Verification items for the finished model (mm, model axes). A direction names the side the tool comes from. Give positions to 0.01 mm unless a question says otherwise; leave off trailing zeros. Order: outer loops, then holes, each group sorted by start corner. A loop starts at its lowest first (then second) coordinate and runs counter-clockwise, first axis right, second up. Notation, with made-up numbers: (31, 68) -> (73, 68) arc R12 cw to (73, 82) -> close; hole circle Ø9 at (82.25, -28.75). An arc over 180 degrees is marked (long way). Return JSON: item names as keys, results as strings. Group by question number.
(1) Cross-section at C-C on y = -6.5. Enter the section's corners in (x, z), then the cut area to 3 significant figures.
(2) Thickness scan on line 1 along Z through (x, y) = (0, -2.25); line 2 along Y through (x, z) = (-5, 5); line 3 along Z through (x, y) = (2.5, -8). Record the ranges inside material, lowest first.
(3) Tool access check on faces 1 (the face through (11.9, -0.5, 2.5)), 2 (the face through (-11.8, -0.5, 2.5)), 3 (the face through (3, -1, 3)), 4 (the face through (11.9, -0.5, -2.5)). Record the directions out of +Z, -Z, +X, -X, +Y, -Y that give a thin tool (end or side, any length) a straight path to the whole face; none if there is none.
(4) Cross-section at A-A on x = 0. Enter the section's corners in (y, z).
(5) Cross-section at B-B on z = 0. Enter the section's corners in (x, y), then the cut area to 3 significant figures.
(6) Cross-section at D-D on z = -8.25. Enter the section's corners in (x, y), then the cut area to 3 significant figures.
(7) Depth check by flat-ended pin: pin 1 Ø4 at (x, y) = (-9, -4) entering from +Z; pin 2 Ø0.8 at (x, y) = (-11.5, -0.5) entering from -Z; pin 3 Ø3 at (y, z) = (-6, -3.5) entering from +X; pin 4 Ø3 at (y, z) = (-2, -8.5) entering from -X. Enter the tip coordinate at first touch or a pass-through.
from build123d import *

# Parameters (mm, degrees)
F0_R          = 11
F1_DEPTH      = 1
F3_W          = 26
F3_H          = 5
F4_DEPTH      = 1
F5_R          = 4
F5_R_2        = 3
F7_DEPTH      = 7.3
F6_R          = 3
F8_DEPTH      = 7.301
F8_DEPTH_BACK = 1.001


with BuildPart() as f1:
    # F0 (on Front) → F1 (new body)
    with BuildSketch(Plane.XZ):
        Circle(F0_R)
    extrude(amount=F1_DEPTH)

    # F3 (on face) → F4 (join)
    with BuildSketch(Plane(origin=(0, 0, 0), x_dir=(-1, 0, 0), z_dir=(0, 1, 0))):
        Rectangle(F3_W, F3_H)
    extrude(amount=-F4_DEPTH)

    # F5 (on face) → F7 (join)
    with BuildSketch(Plane.XZ.offset(1)):
        Circle(F5_R)
        Circle(F5_R_2, mode=Mode.SUBTRACT)
    extrude(amount=F7_DEPTH)

    # F6 (on face) → F8 (cut, two sides)
    with BuildSketch(Plane.XZ.offset(1)) as f8_sk:
        Circle(F6_R)
    extrude(amount=F8_DEPTH, mode=Mode.SUBTRACT)
    extrude(f8_sk.sketch, amount=-F8_DEPTH_BACK, mode=Mode.SUBTRACT)


solid = f1.part
Verdict:
{
 "1": {"outline": "circle Ø8 at (0, 0); hole circle Ø6 at (0, 0)", "area": "22.0 mm²"},
 "2": {"line 1": "-4 to -3, 3 to 4", "line 2": "-1 to 0", "line 3": "-3.12 to -1.66, 1.66 to 3.12"},
 "3": {"face 1": "+Z, +X, +Y, -Y", "face 2": "+Z, -X, +Y, -Y", "face 3": "-Y", "face 4": "-Z, +X, +Y, -Y"},
 "4": {"outline": "(-8.3, -4) -> (-1, -4) -> (-1, -11) -> (0, -11) -> (0, -3) -> (-8.3, -3) -> close; (-8.3, 3) -> (0, 3) -> (0, 11) -> (-1, 11) -> (-1, 4) -> (-8.3, 4) -> close"},
 "5": {"outline": "(-13, -1) -> (-4, -1) -> (-4, -8.3) -> (-3, -8.3) -> (-3, 0) -> (-13, 0) -> close; (3, -8.3) -> (4, -8.3) -> (4, -1) -> (13, -1) -> (13, 0) -> (3, 0) -> close", "area": "34.6 mm²"},
 "6": {"outline": "(-7.28, -1) -> (7.28, -1) -> (7.28, 0) -> (-7.28, 0) -> close", "area": "14.6 mm²"},
 "7": {"pin 1": "through", "pin 2": "z = -2.5", "pin 3": "x = 3.46", "pin 4": "x = -8.16"}
}
